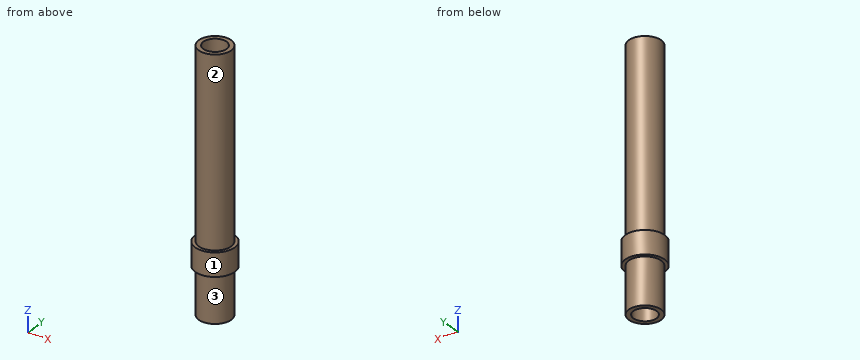
from build123d import *

# Parameters (mm, degrees)
IZIM1_R                     = 3.5
IZIM1_R_2                   = 2.5
Y_KSEKLIK_EKSTR_ZYON1_DEPTH = 50
IZIM2_R                     = 3.5
Y_KSEKLIK_EKSTR_ZYON2_DEPTH = 5
IZIM3_R                     = 4.25
Y_KSEKLIK_EKSTR_ZYON3_DEPTH = 5
IZIM5_R                     = 2.5
KES_EKSTR_ZYON1_DEPTH       = 60


with BuildPart() as part:
    # Çizim1 → Yükseklik-Ekstrüzyon1 (new body)
    with BuildSketch(Plane.XY):
        Circle(IZIM1_R)
        Circle(IZIM1_R_2, mode=Mode.SUBTRACT)
    extrude(amount=Y_KSEKLIK_EKSTR_ZYON1_DEPTH)

    # Çizim2 → Yükseklik-Ekstrüzyon2 (add)
    with BuildSketch(Plane.XY.offset(50)):
        Circle(IZIM2_R)
    extrude(amount=Y_KSEKLIK_EKSTR_ZYON2_DEPTH)

    # Çizim3 → Yükseklik-Ekstrüzyon3 (add)
    with BuildSketch(Plane.XY.offset(10)):
        Circle(IZIM3_R)
    extrude(amount=Y_KSEKLIK_EKSTR_ZYON3_DEPTH)

    # Çizim5 → Kes-Ekstrüzyon1 (cut)
    with BuildSketch(Plane(origin=(0, 0, 10), x_dir=(-1, 0, 0), z_dir=(0, 0, -1))):
        with Locations(Location((0, 0, 0), (0, 0, 180))):
            Circle(IZIM5_R)
    extrude(amount=-KES_EKSTR_ZYON1_DEPTH, mode=Mode.SUBTRACT)


solid = part.part
Could you check a few things on this model? Use its own coordinates, in mm. Face numbers are marked on the shaded views. A direction names the side the tool comes from. Round coordinates to 2 decimals unless told otherwise and drop trailing zeros. Write each loop counter-clockwise with the first axis right and the second up, starting at its lowest first coordinate (ties: lowest second). Pieces come first, ordered by that corner, then holes. Notation, with made-up numbers: (35, 11.25) - (67, 11.25) arc R17 cw to (67, 37.25) - close; hole circle Ø2 at (14.5, 76). An arc over 180 degrees is marked (long way). Put each result on its own line as item: value. Start each with the question number.
(1) I want a section at A-A, the plane x = 0. Please give me the cut outline in (y, z), plus the area to 4 significant figures.
(2) For the marked faces 1, 2 and 3, which set-ups out of +Z, -Z, +X, -X, +Y, -Y let a thin tool reach every point of the face, with its end or its side?
(3) Will these pins go through, and if not, where does the flat tip stop? pin 1 (3 mm diameter, centred on y = -1.5, z = 22, fed in from +X); pin 2 (1 mm diameter, centred on x = 2.5, y = -1.5, fed in from -Z); pin 3 (4 mm diameter, centred on x = 3, z = 20.5, fed in from +Y); pin 4 (4.5 mm diameter, centred on x = 0, y = 0, fed in from -Z).
(4) I need wall thicknesses on probe 1 along Y at (x, z) = (0, 34); probe 2 along X at (y, z) = (-1, 15.5). Which ranges of each line are inside material? Lowest first, please.
(5) I want a section at C-C, the plane z = 23. Please give me the cut outline in (x, y).
Here are the results:
1. outline: (-4.25, 10) - (-3.5, 10) - (-3.5, 0) - (-2.5, 0) - (-2.5, 55) - (-3.5, 55) - (-3.5, 15) - (-4.25, 15) - close; (2.5, 0) - (3.5, 0) - (3.5, 10) - (4.25, 10) - (4.25, 15) - (3.5, 15) - (3.5, 55) - (2.5, 55) - close
1. area: 117.5 mm^2
2. face 1: +Z, -Z
2. face 2: +Z
2. face 3: -Z
3. pin 1: stops at x = 3.5
3. pin 2: stops at z = 0
3. pin 3: stops at y = 3.35
3. pin 4: passes through
4. probe 1: y = -3.5 to -2.5, 2.5 to 3.5
4. probe 2: x = -3.35 to -2.29, 2.29 to 3.35
5. outline: circle Ø7 at (0, 0); hole circle Ø5 at (0, 0)
